Geometry check sheet. Reference: the model listing, model coordinates, mm. Face numbers are marked on the shaded views. Round coordinates to 2 decimals unless told otherwise and drop trailing zeros. Loops run counter-clockwise (first coordinate to the right, second up) from the corner with the lowest first, then second, coordinate; pieces in that order, holes last.
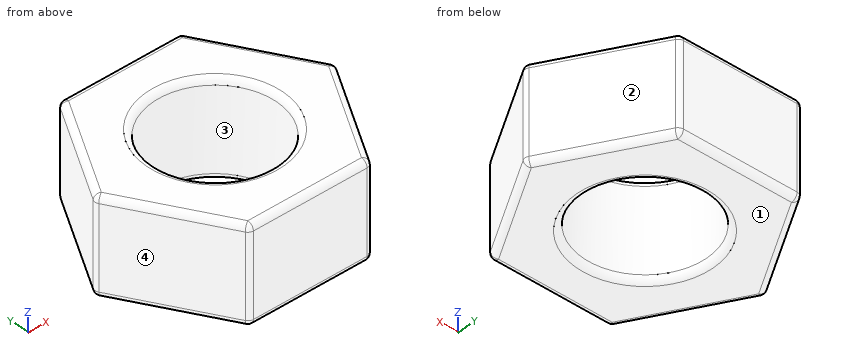
```python
from build123d import *

# Parameters (mm, degrees)
SKIZZE1_R                       = 5
AUFSATZ_LINEAR_AUSTRAGEN1_DEPTH = 3.85
VERRUNDUNG1_R                   = 0.5


with BuildPart() as part:
    # Skizze1 → Aufsatz-Linear austragen1 (new body, symmetric)
    with BuildSketch(Plane.XY):
        Polygon((-9.814954576, 0), (-4.907477288, -8.5), (4.907477288, -8.5), (9.814954576, 0), (4.907477288, 8.5), (-4.907477288, 8.5), align=None)
        Circle(SKIZZE1_R, mode=Mode.SUBTRACT)
    extrude(amount=AUFSATZ_LINEAR_AUSTRAGEN1_DEPTH, both=True)

    # Verrundung1
    verrundung1_edges = [part.edges().sort_by_distance(p)[0] for p in [
        (-4.907477288, 8.5, 0),
        (4.907477288, 8.5, 0),
        (9.814954576, 0, 0),
        (4.907477288, -8.5, 0),
        (-4.907477288, -8.5, 0),
        (-9.814954576, 0, 0),
        (0, -8.5, 3.85),
        (7.361215932, -4.25, 3.85),
        (-5, 0, -3.85),
        (-5, 0, 3.85),
        (7.361215932, 4.25, 3.85),
        (0, 8.5, 3.85),
        (-7.361215932, 4.25, 3.85),
        (0, 8.5, -3.85),
        (7.361215932, 4.25, -3.85),
        (7.361215932, -4.25, -3.85),
        (0, -8.5, -3.85),
        (-7.361215932, -4.25, -3.85),
        (-7.361215932, 4.25, -3.85),
        (-7.361215932, -4.25, 3.85),
    ]]
    fillet(verrundung1_edges, radius=VERRUNDUNG1_R)


solid = part.part
```
1) Scan lines: line 1 along Y through (x, z) = (0, 1.5); line 2 along Y through (x, z) = (-2.25, -3); line 3 along X through (y, z) = (-0.75, 0). Record each from-to range of solid material in increasing order.
Report:
line 1: y = -8.5 to -5, 5 to 8.5
line 2: y = -8.5 to -4.47, 4.47 to 8.5
line 3: x = -9.38 to -4.94, 4.94 to 9.38
2) Sectioned sample at A-A, the plane x = 0. Record the cut outline in (y, z).
Report:
outline: (-8.5, -3.35) arc R0.5 ccw to (-8, -3.85) - (-5.5, -3.85) arc R0.5 ccw to (-5, -3.35) - (-5, 3.35) arc R0.5 ccw to (-5.5, 3.85) - (-8, 3.85) arc R0.5 ccw to (-8.5, 3.35) - close; (5, -3.35) arc R0.5 ccw to (5.5, -3.85) - (8, -3.85) arc R0.5 ccw to (8.5, -3.35) - (8.5, 3.35) arc R0.5 ccw to (8, 3.85) - (5.5, 3.85) arc R0.5 ccw to (5, 3.35) - close
3) Gauge pin test, flat ends, axial feed: pin 1 (1.5 mm diameter, centred on x = 0, y = 3, fed in from +Z); pin 2 (4 mm diameter, centred on y = -6.5, z = -2, fed in from +X); pin 3 (5 mm diameter, centred on x = -3.5, y = -2, fed in from -Z). Record the tip position at first contact, or that the pin passes through.
Report:
pin 1: passes through
pin 2: stops at x = 7.22
pin 3: stops at z = -3.85
4) Mould release check, pull along Y, two halves, no side actions. Record for the marked faces 1, 2, 3 and 4: +Y half, -Y half, draft (parallel to the pull), parting line (faces both ways), or undercut.
Report:
face 1: draft
face 2: +Y half
face 3: undercut
face 4: -Y half
5) Sectioned sample at B-B, the plane z = 0.25. Record the cut outline in (x, y).
Report:
outline: (-9.67, -0.25) - (-5.05, -8.25) arc R0.5 ccw to (-4.62, -8.5) - (4.62, -8.5) arc R0.5 ccw to (5.05, -8.25) - (9.67, -0.25) arc R0.5 ccw to (9.67, 0.25) - (5.05, 8.25) arc R0.5 ccw to (4.62, 8.5) - (-4.62, 8.5) arc R0.5 ccw to (-5.05, 8.25) - (-9.67, 0.25) arc R0.5 ccw to start; hole circle Ø10 at (0, 0)
